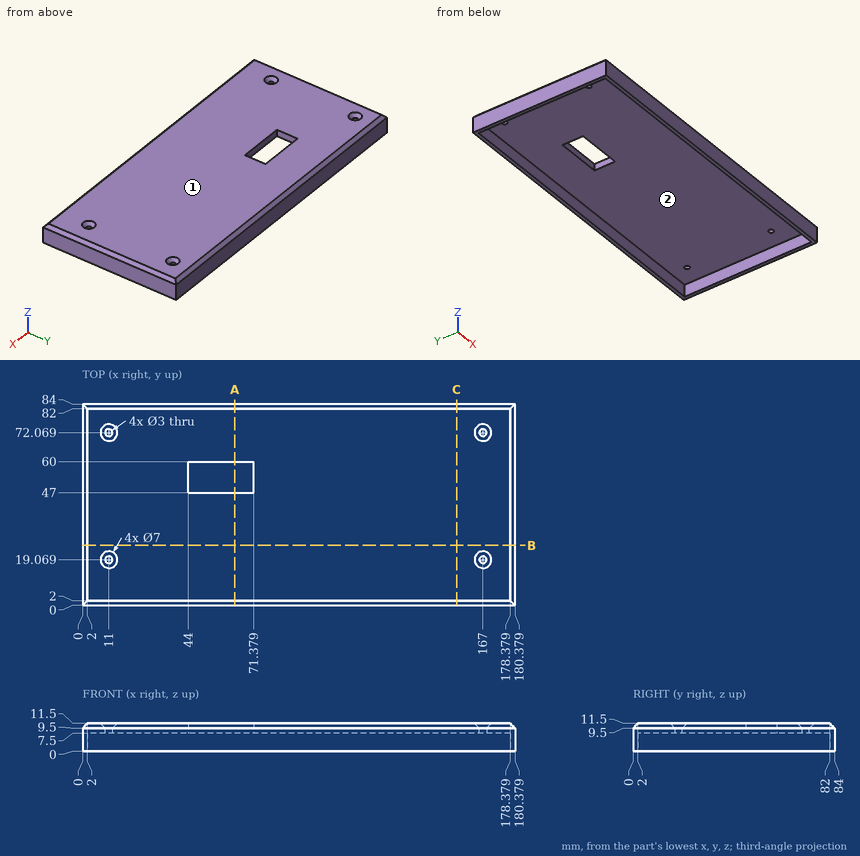
For this review, use the dimensioned drawing (mm, ordinates from the lowest corner) and the shaded views. Round coordinates to 2 decimals unless told otherwise and drop trailing zeros. Write each loop counter-clockwise with the first axis right and the second up, starting at its lowest first coordinate (ties: lowest second). Pieces come first, ordered by that corner, then holes. Notation, with made-up numbers: (55, 1.25) -> (84, 1.25) arc R28 cw to (84, 28.25) -> close; hole circle Ø3 at (60.25, -18). An arc over 180 degrees is marked (long way). One line per item, written item: value. Start each with the question number.
Q1. Add section B-B (y = 25). Give the boundary of the cut face in (x, z).
Q2. Add section A-A (x = 63.5). Give the boundary of the cut face in (y, z), then the cut area to 3 significant figures.
Q3. To check wall thickness, follow probe 1 along Y at (x, z) = (167, 8.1); probe 2 along Y at (x, z) = (144.5, 1.5); probe 3 along X at (y, z) = (33, 4.5). State the ranges of each line that lie inside material, in increasing order.
Q4. The part is to be moulded in two halves that separate along Y. For the marked faces 1 and 2, say which applies: pulls with the +Y half, pulls with the -Y half, needs draft (parallel to the pull), parting line crosses it, or undercut.
Q5. Insertion check: P1, Ø2.5, axis at x = 11, y = 19.07, coming from the -Z side; P2, Ø24, axis at x = 118.5, y = 25, coming from the -Z side. Each pin has a flat end and moves straight along its axis. Give the tip position at first contact, or say it passes through.
Q6. Add section C-C (x = 156). Give the boundary of the cut face in (y, z).
Response:
1. outline: (0, 0) -> (2, 0) -> (2, 7.5) -> (178.38, 7.5) -> (178.38, 0) -> (180.38, 0) -> (180.38, 9.5) -> (178.38, 11.5) -> (2, 11.5) -> (0, 9.5) -> close
2. outline: (0, 0) -> (2, 0) -> (2, 7.5) -> (47, 7.5) -> (47, 11.5) -> (2, 11.5) -> (0, 9.5) -> close; (60, 7.5) -> (82, 7.5) -> (82, 0) -> (84, 0) -> (84, 9.5) -> (82, 11.5) -> (60, 11.5) -> close
2. area: 310 mm^2
3. probe 1: y = 0 to 17.57, 20.57 to 70.57, 73.57 to 84
3. probe 2: y = 0 to 2, 82 to 84
3. probe 3: x = 0 to 2, 178.38 to 180.38
4. face 1: needs draft
4. face 2: undercut
5. P1: passes through
5. P2: stops at z = 7.5
6. outline: (0, 0) -> (2, 0) -> (2, 7.5) -> (82, 7.5) -> (82, 0) -> (84, 0) -> (84, 9.5) -> (82, 11.5) -> (2, 11.5) -> (0, 9.5) -> close
